For this review, take the finished solid that the model builds, in its own axes (mm). A direction names the side the tool comes from. Coordinates: 2 decimals unless noted, no trailing zeros. Loops run counter-clockwise (first coordinate to the right, second up) from the corner with the lowest first, then second, coordinate; pieces in that order, holes last. Notation, with made-up numbers: M -16,68.25 L 8,68.25 A27 cw 8,96.25 Z; hole C 76.5,71.25 d10. An arc over 180 degrees is marked long. Answer as a JSON object with one key per item and string values. Group by question number.
Item 1: Mouldability with a two-part tool opening along X and no side actions: class faces 4 (the face through (-50, -31, 10)), 5 (the face through (5.5, -39.88, -0.05)), 6 (the face through (-8.85, -67.42, -0.14)) as +X half, -X half, draft (parallel to the pull), parting line (faces both ways), or undercut.
Item 2: Insertion check: pin 1 (19.5 mm diameter, centred on x = -45.18, y = -14.68, fed in from -Z); pin 2 (3 mm diameter, centred on y = -51.5, z = -6, fed in from -X); pin 3 (1 mm diameter, centred on y = 11, z = 7.5, fed in from -X); pin 4 (13 mm diameter, centred on x = 0, y = 0, fed in from -Z). Each pin has a flat end and moves straight along its axis. Give the tip position at first contact, or say it passes through.
Item 3: Tool access review of faces 1 (the face through (26.76, 51.46, 6.8)), 2 (the face through (-1.63, -54.82, -0.05)), 3 (the face through (11.923, -3.755, -6.796)): name each direction out of +Z, -Z, +X, -X, +Y, -Y from which nothing blocks a thin tool from reaching the whole face with its end or side.
Item 4: Add section A-A (z = -5.75). State the section outline as (x, y) points, then the cut area to 3 significant figures.
Item 5: Add section B-B (x = 0). Count the separate pieces of the cut face and the enclosed holes in it, then the cut area to 3 significant figures.
Item 6: Add section C-C (y = 25.5). State the section outline as (x, z) points, then the cut area to 3 significant figures.
Item 7: Add section D-D (x = 42.5). State the section outline as (y, z) points, then the cut area to 3 significant figures.
Item 8: Wall thickness on L1, parallel to Y at x = 0, z = 1; L2, parallel to X at y = -6, z = 6; L3, parallel to X at y = 31.5, z = -3.25: over which ranges is each line inside the solid? List them lowest first. Write a range as from..to.
from build123d import *

# Parameters (mm, degrees)
CUT_EXTRUDE1_DEPTH      = 97.685055722
CUT_EXTRUDE1_DEPTH_BACK = 97.685055722
SKETCH2_R               = 7.5
SKETCH2_R_2             = 19


with BuildPart() as part:
    # Sketch1 → Revolve1 (revolve)
    with BuildSketch(Plane(origin=(0, 0, 0), x_dir=(0, 0, -1), z_dir=(1, 0, 0)), mode=Mode.PRIVATE) as revolve1_sk:
        Polygon((-10, 68), (10, 68), (10, 58), (3.5, 58), (3.5, 12.5), (10, 12.5), (10, 4), (-10, 4), (-10, 12.5), (-3.5, 12.5), (-3.5, 58), (-10, 58), align=None)
    revolve(revolve1_sk.sketch.rotate(Axis((0, 0, 51.457627119), (0, 0, -1)), 90), axis=Axis((0, 0, 51.457627119), (0, 0, -1)))

    # Sketch2 → Cut-Extrude1 (cut, two sides: drawn at the far end of the back side and taken through both)
    with BuildSketch(Plane.XY.offset(-CUT_EXTRUDE1_DEPTH_BACK)):
        with Locations((0, -47.5)):
            Circle(SKETCH2_R)
        with Locations((45.175184524, -14.678307233)):
            Circle(SKETCH2_R)
        with Locations((27.919799484, 38.428307233)):
            Circle(SKETCH2_R)
        with Locations((-27.919799484, 38.428307233)):
            Circle(SKETCH2_R)
        with Locations((-45.175184524, -14.678307233)):
            Circle(SKETCH2_R)
        with Locations((0, 35)):
            Circle(SKETCH2_R_2)
        with Locations((33.287669053, 10.81654586)):
            Circle(SKETCH2_R_2)
        with Locations((20.574292847, -28.315007018)):
            Circle(SKETCH2_R_2)
        with Locations((-20.570674813, -28.316182588)):
            Circle(SKETCH2_R_2)
        with Locations((-33.286287087, 10.814643747)):
            Circle(SKETCH2_R_2)
    extrude(amount=CUT_EXTRUDE1_DEPTH + CUT_EXTRUDE1_DEPTH_BACK, mode=Mode.SUBTRACT)


solid = part.part
From the geometry:
{
 "1": {"face 4": "draft", "face 5": "undercut", "face 6": "parting line"},
 "2": {"pin 1": "stops at z = -3.5", "pin 2": "stops at x = -46.09", "pin 3": "stops at x = -67.18", "pin 4": "stops at z = -10"},
 "3": {"face 1": "+Z", "face 2": "+Z, -Z", "face 3": "-Z"},
 "4": {"outline": "C 0,0 d136; C 0,0 d25; hole C 0,0 d116; hole C 0,0 d8", "area": "4,400 mm²"},
 "5": {"separate pieces": "4", "enclosed holes": "0", "area": "1,010 mm²"},
 "6": {"outline": "M -63.04,-10 L -52.09,-10 L -52.09,-3.5 L -45.34,-3.5 L -45.34,3.5 L -52.09,3.5 L -52.09,10 L -63.04,10 Z; M -21.23,-3.5 L -16.45,-3.5 L -16.45,3.5 L -21.23,3.5 Z; M 16.45,-3.5 L 21.23,-3.5 L 21.23,3.5 L 16.45,3.5 Z; M 45.35,-3.5 L 52.09,-3.5 L 52.09,-10 L 63.04,-10 L 63.04,10 L 52.09,10 L 52.09,3.5 L 45.35,3.5 Z", "area": "599 mm²"},
 "7": {"outline": "M -53.08,-10 L -39.47,-10 L -39.47,-3.5 L -21.68,-3.5 L -21.68,3.5 L -39.47,3.5 L -39.47,10 L -53.08,10 Z; M -7.67,-3.5 L -5.8,-3.5 L -5.8,3.5 L -7.67,3.5 Z; M 27.43,-3.5 L 39.47,-3.5 L 39.47,-10 L 53.08,-10 L 53.08,10 L 39.47,10 L 39.47,3.5 L 27.43,3.5 Z", "area": "766 mm²"},
 "8": {"L1": "y = -68..-55, -40..-4, 4..16, 54..68", "L2": "x = -67.73..-57.69, -10.97..10.97, 57.69..67.73", "L3": "x = -60.26..-30.79, -25.05..-18.67, 18.67..25.05, 30.79..60.26"}
}
